```python
from build123d import *

# Parameters (mm, degrees)
SKETCH1_W           = 100
SKETCH1_H           = 100
BOSS_EXTRUDE1_DEPTH = 30
CUT_EXTRUDE1_DEPTH  = 31


with BuildPart() as part:
    # Sketch1 → Boss-Extrude1 (new body)
    with BuildSketch(Plane(origin=(0, 0, 0), x_dir=(1, 0, 0), z_dir=(0, 1, 0))):
        Rectangle(SKETCH1_W, SKETCH1_H)
    extrude(amount=BOSS_EXTRUDE1_DEPTH)

    # Sketch2 → Cut-Extrude1 (cut, through all)
    with BuildSketch(Plane(origin=(0, 30, 0), x_dir=(1, 0, 0), z_dir=(0, 1, 0))):
        Polygon((40, 40), (40, -40), (-40, -40), align=None)
    extrude(amount=-CUT_EXTRUDE1_DEPTH, mode=Mode.SUBTRACT)


solid = part.part
```
The listing builds one solid part. Answer for the finished solid, in the listing's coordinates (mm). A direction names the side the tool comes from. Give positions to 0.01 mm unless a question says otherwise; leave off trailing zeros. Loops run counter-clockwise (first coordinate to the right, second up) from the corner with the lowest first, then second, coordinate; pieces in that order, holes last. Notation, with made-up numbers: M 28,-17.75 L 35,-17.75 A28 ccw 35,0.25 Z; hole C -15,18.25 d9. An arc over 180 degrees is marked long. One line per item, written item: value.
Q1. Find the intervals of material crossed by line 1 (X direction, y = 27, z = 2); line 2 (X direction, y = 27.5, z = 31.5); line 3 (Z direction, x = 36, y = 9.5), in increasing order. Write a range as from..to.
Working result:
line 1: x = -50..-2, 40..50
line 2: x = -50..-31.5, 40..50
line 3: z = -50..-36, 40..50
Q2. For faces 1 (the face through (-1, 30, -1)), 2 (the face through (40, 15, -1)), determine the directions among +Z, -Z, +X, -X, +Y, -Y from which every point of the face is accessible in a straight line to the end or side of a thin tool.
Working result:
face 1: +Z, -Z, +X, -X, +Y
face 2: +Y, -Y
Q3. Determine the mould class of faces 3 (the face through (-1, 15, 1)), 4 (the face through (-1, 15, -50)), 5 (the face through (1, 15, 40)), 6 (the face through (50, 15, 1)) for opening direction Z: +Z half, -Z half, draft (parallel to the pull), parting line (faces both ways), or undercut.
Working result:
face 3: undercut
face 4: -Z half
face 5: undercut
face 6: draft
Q4. A cutting plane is placed at A-A on z = -1.5. Determine the outline of the cut face in (x, y).
Working result:
outline: M -50,0 L 1.5,0 L 1.5,30 L -50,30 Z; M 40,0 L 50,0 L 50,30 L 40,30 Z
Q5. A cutting plane is placed at B-B on x = 23. Determine the outline of the cut face in (y, z), then the cut area to 3 significant figures.
Working result:
outline: M 0,-50 L 30,-50 L 30,-23 L 0,-23 Z; M 0,40 L 30,40 L 30,50 L 0,50 Z
area: 1,110 mm^2
Q6. A cutting plane is placed at C-C on y = 18. Determine the outline of the cut face in (x, z).
Working result:
outline: M -50,-50 L 50,-50 L 50,50 L -50,50 Z; hole M -40,40 L 40,-40 L 40,40 Z
